from build123d import *

# Parameters (mm, degrees)
SKETCH1_R           = 1
SKETCH1_R_2         = 24.607140245
BOSS_EXTRUDE1_DEPTH = 0.25


with BuildPart() as part:
    # Sketch1 → Boss-Extrude1 (new body)
    with BuildSketch(Plane(origin=(0, 0, 0), x_dir=(1, 0, 0), z_dir=(0, 1, 0))):
        with BuildLine():
            Line((-26.75, 11.088438625), (-26.75, -11.088438625))
            ThreePointArc((-26.75, -11.088438625), (0, -28.957140245), (26.75, -11.088438625))
            Line((26.75, -11.088438625), (26.75, 11.088438625))
            ThreePointArc((26.75, 11.088438625), (0, 28.957140245), (-26.75, 11.088438625))
        make_face()
        with Locations(Location((18.839877725, -18.839877725, 0), (0, 0, 270))):
            Circle(SKETCH1_R, mode=Mode.SUBTRACT)
        with Locations(Location((18.839877725, 18.839877725, 0), (0, 0, 270))):
            Circle(SKETCH1_R, mode=Mode.SUBTRACT)
        with Locations(Location((-18.839877725, 18.839877725, 0), (0, 0, 270))):
            Circle(SKETCH1_R, mode=Mode.SUBTRACT)
        with Locations(Location((-18.839877725, -18.839877725, 0), (0, 0, 270))):
            Circle(SKETCH1_R, mode=Mode.SUBTRACT)
        with Locations(Location((0, 0, 0), (0, 0, 270))):
            Circle(SKETCH1_R_2, mode=Mode.SUBTRACT)
    extrude(amount=BOSS_EXTRUDE1_DEPTH)


solid = part.part
Can you work these out from the model? Positions are in its coordinate system, mm. Coordinates: 2 decimals unless noted, no trailing zeros. Order: outer loops, then holes, each group sorted by start corner. A loop starts at its lowest first (then second) coordinate and runs counter-clockwise, first axis right, second up. Notation, with made-up numbers: M -4.5,87.5 L 1.5,87.5 A13 ccw 1.5,112.5 Z; hole C 31,30.5 d7. An arc over 180 degrees is marked long. Write item = value, one per line.
(1) I need wall thicknesses on line 1 along Z through (x, y) = (18, 0.1); line 2 along X through (y, z) = (0.1, 0). Which ranges of each line are inside material? Lowest first, please. Write a range as [from, to].
Results are:
line_1 = [-22.68, -19.38], [-18.3, -16.78], [16.78, 18.3], [19.38, 22.68]
line_2 = [-26.75, -24.61], [24.61, 26.75]
(2) Suppose I cut it at B-B on x = 12.5. Please give me the cut outline in (y, z).
Results are:
outline = M 0,-26.12 L 0.25,-26.12 L 0.25,-21.2 L 0,-21.2 Z; M 0,21.2 L 0.25,21.2 L 0.25,26.12 L 0,26.12 Z
(3) For pin 1 Ø1.6 at (x, z) = (18.84, -18.84) entering from +Y, with a flat end and sliding along its axis, tell me the tip position at first contact or that it passes through.
Results are:
pin_1 = through
(4) Suppose I cut it at A-A on z = 0. Please give me the cut outline in (x, y).
Results are:
outline = M -26.75,0 L -24.61,0 L -24.61,0.25 L -26.75,0.25 Z; M 24.61,0 L 26.75,0 L 26.75,0.25 L 24.61,0.25 Z
(5) Suppose I cut it at C-C on y = 0.1. Please give me the cut outline in (x, z), plus the area to 3 significant figures.
Results are:
outline = M -26.75,-11.09 A28.96 ccw 26.75,-11.09 L 26.75,11.09 A28.96 ccw -26.75,11.09 Z; hole C 0,0 d49.21; hole C -18.84,-18.84 d2; hole C -18.84,18.84 d2; hole C 18.84,-18.84 d2; hole C 18.84,18.84 d2
area = 654 mm2
